Geometry: see drawing. Coordinates: mm, zero at the bounding-box minimum. A direction names the side the tool comes from. Round coordinates to 2 decimals unless told otherwise and drop trailing zeros. Order: outer loops, then holes, each group sorted by start corner. A loop starts at its lowest first (then second) coordinate and runs counter-clockwise, first axis right, second up. Notation, with made-up numbers: (10, 55) -> (55, 55) arc R16 cw to (55, 71) -> close; hole circle Ø7 at (42.5, -37.5). An arc over 180 degrees is marked (long way). Put each result on its own line as item: value.
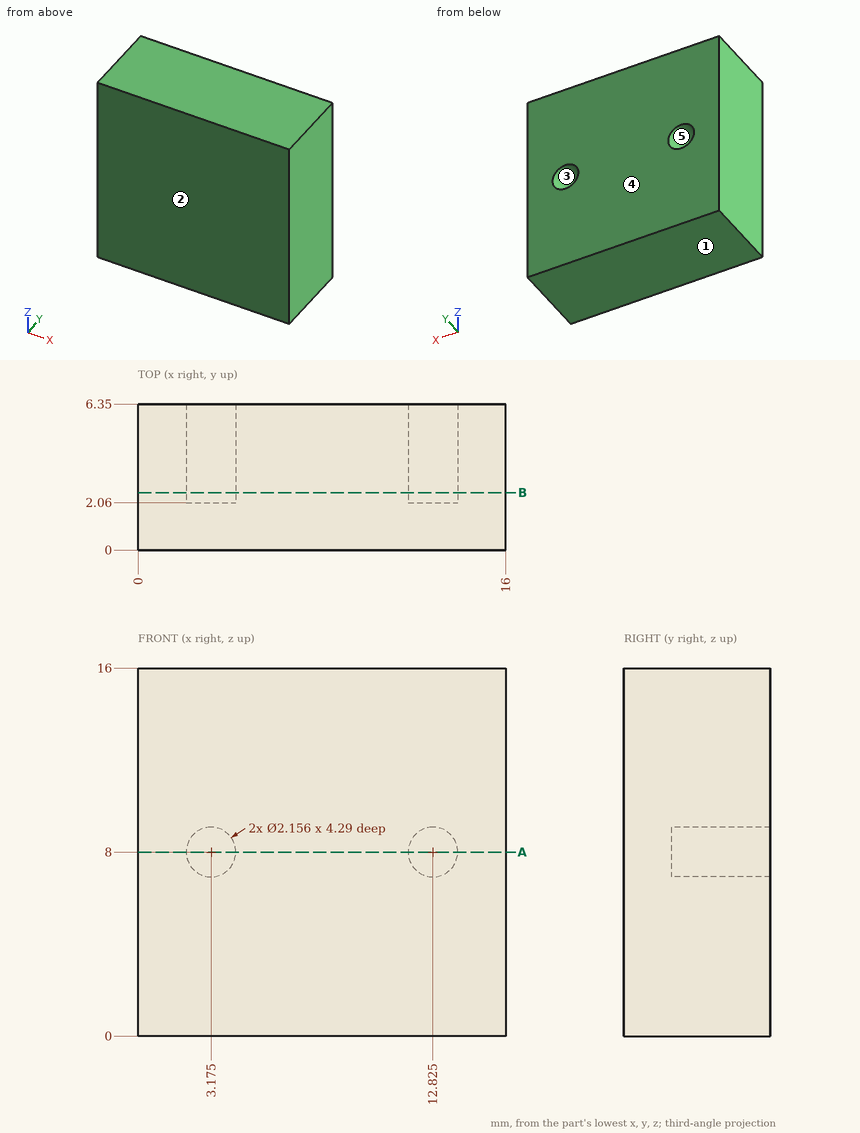
1. Cut plane A-A on z = 8. Return loops of the section in (x, y).
Ans:
outline: (0, 0) -> (16, 0) -> (16, 6.35) -> (13.9, 6.35) -> (13.9, 2.06) -> (11.75, 2.06) -> (11.75, 6.35) -> (4.25, 6.35) -> (4.25, 2.06) -> (2.1, 2.06) -> (2.1, 6.35) -> (0, 6.35) -> close
2. Draft query along Z for the marked faces 1, 2 and 3. Return one class per face: +Z half, -Z half, draft (parallel to the pull), parting line (faces both ways), or undercut.
Ans:
face 1: -Z half
face 2: draft
face 3: undercut
3. Cut plane B-B on y = 2.5. Return loops of the section in (x, z) (1 decimal), and give its area (3 significant figures).
Ans:
outline: (0, 0) -> (16, 0) -> (16, 16) -> (0, 16) -> close; hole circle Ø2.2 at (3.2, 8); hole circle Ø2.2 at (12.8, 8)
area: 249 mm²
4. Material intervals for probe 1 along X at (y, z) = (3.7, 8); probe 2 along Z at (x, y) = (2.75, 3.25); probe 3 along Z at (x, y) = (13, 4.5) (1 decimal), sorted ascending.
Ans:
probe 1: 0 to 2.1, 4.25 to 11.75, 13.9 to 16
probe 2: 0 to 7.01, 8.99 to 16
probe 3: 0 to 6.9, 9.1 to 16
5. Contact query for flat-ended pins moving along their axis: P1, Ø2, axis at y = 2, z = 7, coming from the -X side; P2, Ø0.6, axis at x = 3.5, z = 7.5, coming from the +Y side. Output: stop coordinate, or through.
Ans:
P1: x = 0
P2: y = 2.06
6. Set-up query: the marked faces 4 and 5. Return all of +Z, -Z, +X, -X, +Y, -Y with unobstructed straight access to the full face (end or side cutting, diameter ignored); none if empty.
Ans:
face 4: +Z, -Z, +X, -X, +Y
face 5: +Y
